Answer from the drawing. Dimensions are ordinates in mm from the lowest x, y and z of the part. A direction names the side the tool comes from. Give positions to 0.01 mm unless a question says otherwise; leave off trailing zeros. Write each loop counter-clockwise with the first axis right and the second up, starting at its lowest first coordinate (ties: lowest second). Pieces come first, ordered by that corner, then holes. Notation, with made-up numbers: M -28,28 L 0,28 A24 ccw 0,49 Z; hole C -25.75,18.25 d9. An arc over 180 degrees is marked long. Put each result on its own line as item: value.
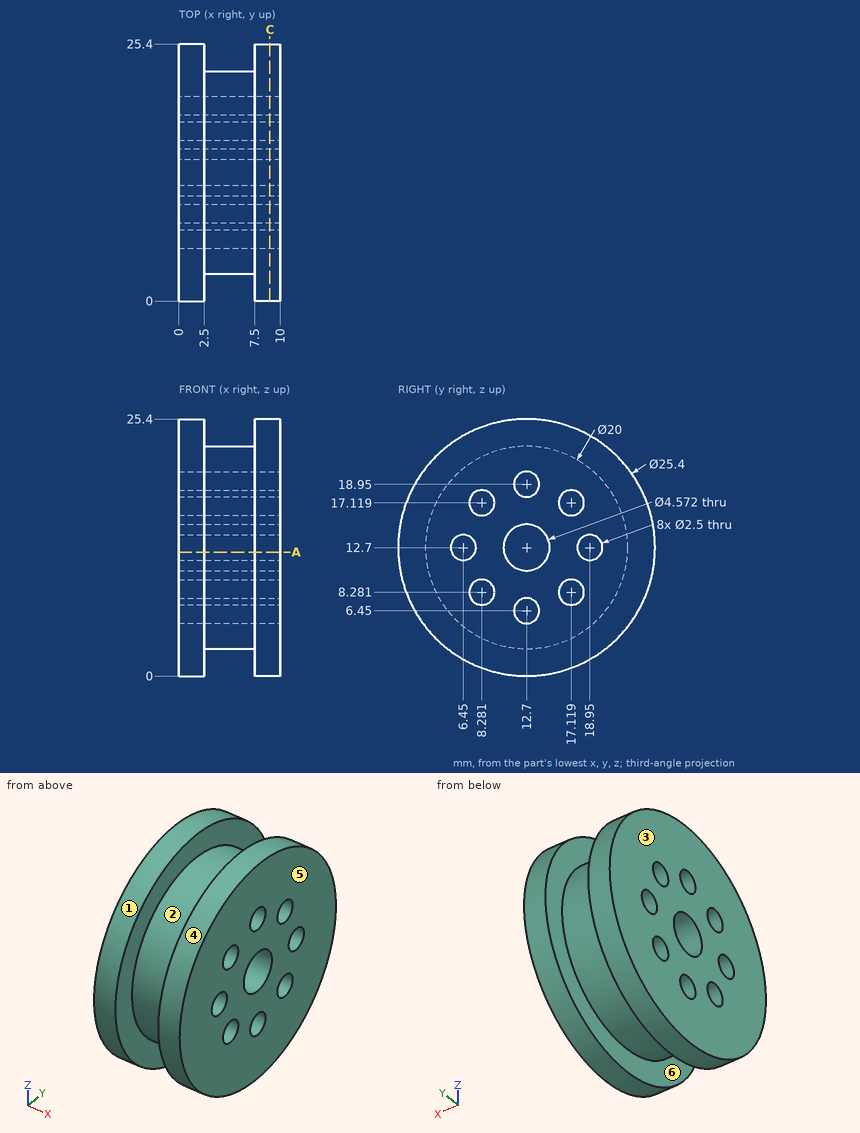
(1) Section C-C on x = 9 is taken. Give the number of separate pieces and of enclosed holes in the cut face, and give its area (3 significant figures).
Result:
separate pieces: 1
enclosed holes: 9
area: 451 mm²
(2) For a pull along X with two mould halves and no side action, classify the marked faces 3, 4, 5 and 6 as +X half, -X half, draft (parallel to the pull), parting line (faces both ways), or undercut.
Result:
face 3: -X half
face 4: draft
face 5: +X half
face 6: undercut
(3) Section A-A on z = 12.25 is taken. Determine the outline of the cut face in (x, y).
Result:
outline: M 0,0.01 L 2.5,0.01 L 2.5,2.71 L 7.5,2.71 L 7.5,0.01 L 10,0.01 L 10,5.28 L 0,5.28 Z; M 0,7.62 L 10,7.62 L 10,10.46 L 0,10.46 Z; M 0,14.94 L 10,14.94 L 10,17.78 L 0,17.78 Z; M 0,20.12 L 10,20.12 L 10,25.39 L 7.5,25.39 L 7.5,22.69 L 2.5,22.69 L 2.5,25.39 L 0,25.39 Z
(4) Straight lines are drawn through the part: line 1 along Z through (x, y) = (5.5, 12.7); line 2 along X through (y, z) = (2, 12); line 3 along Z through (x, y) = (9, 16) (1 decimal). For each, find the intervals that lie inside material, in ascending order. Write a range as from..to.
Result:
line 1: z = 2.7..5.2, 7.7..10.41, 14.99..17.7, 20.2..22.7
line 2: x = 0..2.5, 7.5..10
line 3: z = 0.4..7.7, 8.8..16.6, 17.7..25
(5) Which of the six approach directions +Z, -Z, +X, -X, +Y, -Y give full straight-line access (tool end or side, diameter ignored) to the marked faces 1 and 2?
Result:
face 1: +X, -X
face 2: none
(6) Given pin 1 Ø2 at (y, z) = (17.12, 8.28) entering from +X; pin 2 Ø6 at (x, z) = (2.5, 20.5) entering from +Y; pin 3 Ø1.5 at (x, z) = (7.5, 18.5) entering from -Y; pin 4 Ø1.5 at (x, z) = (4.5, 5) entering from -Y, each flat-ended and moving along its own axis, determine where each tip first touches the part or whether it passes through.
Result:
pin 1: passes through
pin 2: stops at y = 24.46
pin 3: stops at y = 1.05
pin 4: stops at y = 5.51
